Source: CAD feature listing. Evaluate the final solid. Frame: model axes, mm. Face numbers are marked on the shaded views. A direction names the side the tool comes from. Coordinates: 2 decimals unless noted, no trailing zeros. Order: outer loops, then holes, each group sorted by start corner. A loop starts at its lowest first (then second) coordinate and runs counter-clockwise, first axis right, second up.
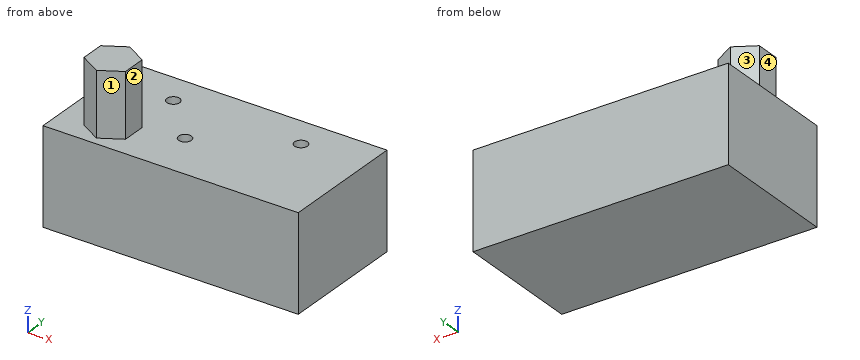
```python
from build123d import *

# Parameters (mm, degrees)
F0_W     = 101.6
F0_H     = 50.8
F1_DEPTH = 38.1
F3_D     = 5.1054
F3_DEPTH = 16.51
F3_TIP   = 1.5338169022
F5_DEPTH = 25.4


with BuildPart() as f1:
    # F0 (on Top) → F1 (new body)
    with BuildSketch(Plane.XY):
        with Locations((50.8, -25.4)):
            Rectangle(F0_W, F0_H)
    extrude(amount=F1_DEPTH)

    # F3
    with Locations(Plane.XY.offset(38.1)):
        with Locations((25.4, -12.7), (42.8625, -31.1450831863), (76.2, -12.7)):
            Hole(F3_D / 2, depth=F3_DEPTH)
            with Locations((0, 0, -(F3_DEPTH + F3_TIP / 2))):  # 118° drill point
                Cone(0, F3_D / 2, F3_TIP, mode=Mode.SUBTRACT)

    # F4 (on face) → F5 (join)
    with BuildSketch(Plane.XY.offset(38.1)):
        Polygon((19.05, -47.625), (27.298891971, -42.8625), (27.298891971, -33.3375), (19.05, -28.575), (10.801108029, -33.3375), (10.801108029, -42.8625), align=None)
    extrude(amount=F5_DEPTH)


solid = f1.part
```
Q1. Material intervals for line 1 along X through (y, z) = (-12.7, 31.5); line 2 along Y through (x, z) = (76.2, 29.75); line 3 along X through (y, z) = (-12, 31), sorted ascending.
Solutions:
line 1: x = 0 to 22.85, 27.95 to 73.65, 78.75 to 101.6
line 2: y = -50.8 to -15.25, -10.15 to 0
line 3: x = 0 to 22.95, 27.85 to 73.75, 78.65 to 101.6
Q2. Section query C-C on x = 37. Output: boundary loops of the cut face in (y, z).
Solutions:
outline: (-50.8, 0) - (0, 0) - (0, 38.1) - (-50.8, 38.1) - close
Q3. Pin query (flat end, axial travel): P1, Ø4.5, axis at x = 76.2, y = -12.7, coming from the +Z side; P2, Ø10.5, axis at y = -39, z = 47.5, coming from the -X side; P3, Ø6, axis at y = -19, z = 42.5, coming from the +X side; P4, Ø12, axis at x = 27, z = 57, coming from the -Y side. Return the tip coordinate at first contact, or that it passes through.
Solutions:
P1: stops at z = 21.41
P2: stops at x = 10.8
P3: passes through
P4: stops at y = -46.5
Q4. Section query B-B on y = -26. Output: boundary loops of the cut face in (x, z), plus the area to 3 significant figures.
Solutions:
outline: (0, 0) - (101.6, 0) - (101.6, 38.1) - (0, 38.1) - close
area: 3,870 mm2
Q5. Set-up query: the marked faces 1, 2, 3 and 4. Return all of +Z, -Z, +X, -X, +Y, -Y with unobstructed straight access to the full face (end or side cutting, diameter ignored); none if empty.
Solutions:
face 1: +Z, +X, -Y
face 2: +Z, +X, +Y, -Y
face 3: +Z, -X, +Y
face 4: +Z, -X, +Y, -Y
